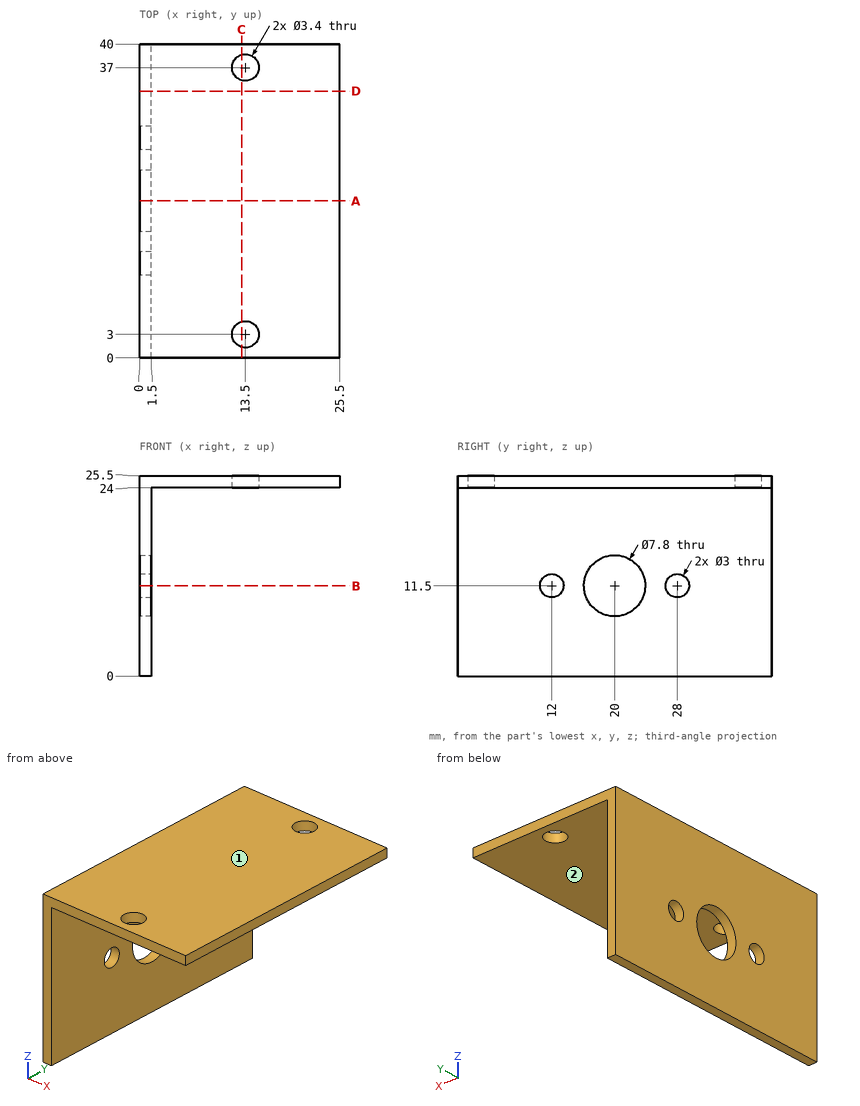
The drawing under review shows one solid part. Ordinate dimensions are in mm from its lowest x, y, z. A direction names the side the tool comes from. Round coordinates to 2 decimals unless told otherwise and drop trailing zeros. Write each loop counter-clockwise with the first axis right and the second up, starting at its lowest first coordinate (ties: lowest second). Pieces come first, ordered by that corner, then holes. Notation, with made-up numbers: (63, 58.25) - (115, 58.25) arc R16 cw to (115, 81.25) - close; hole circle Ø8 at (-4.5, 49.25). An arc over 180 degrees is marked (long way). One line per question, with ' | ' between items.
Item 1: For P1, Ø9, axis at y = 20, z = 11.5, coming from the +X side; P2, Ø1.5, axis at x = 13, y = 21.5, coming from the -Z side; P3, Ø10, axis at x = 9.5, z = 11.5, coming from the -Y side, all flat-tipped, find the tip position at first contact; note any pin that passes through.
Resolved:
P1: stops at x = 1.5 | P2: stops at z = 24 | P3: passes through
Item 2: Add section C-C, the plane x = 13. Give the boundary of the cut face in (y, z).
Resolved:
outline: (0, 24) - (1.38, 24) - (1.38, 25.5) - (0, 25.5) - close; (4.62, 24) - (35.38, 24) - (35.38, 25.5) - (4.62, 25.5) - close; (38.62, 24) - (40, 24) - (40, 25.5) - (38.62, 25.5) - close
Item 3: To check wall thickness, follow probe 1 along Y at (x, z) = (13.5, 24.7); probe 2 along Y at (x, z) = (0.8, 11.5); probe 3 along X at (y, z) = (29.5, 12.25). State the ranges of each line that lie inside material, in increasing order.
Resolved:
probe 1: y = 0 to 1.3, 4.7 to 35.3, 38.7 to 40 | probe 2: y = 0 to 10.5, 13.5 to 16.1, 23.9 to 26.5, 29.5 to 40 | probe 3: x = 0 to 1.5
Item 4: Add section D-D, the plane y = 34. Give the boundary of the cut face in (x, z), then the cut area to 4 significant figures.
Resolved:
outline: (0, 0) - (1.5, 0) - (1.5, 24) - (25.5, 24) - (25.5, 25.5) - (0, 25.5) - close | area: 74.25 mm2
Item 5: Add section A-A, the plane y = 20. Give the boundary of the cut face in (x, z), then the cut area to 4 significant figures.
Resolved:
outline: (0, 0) - (1.5, 0) - (1.5, 7.6) - (0, 7.6) - close; (0, 15.4) - (1.5, 15.4) - (1.5, 24) - (25.5, 24) - (25.5, 25.5) - (0, 25.5) - close | area: 62.55 mm2
Item 6: Add section B-B, the plane z = 11.5. Give the boundary of the cut face in (x, y), then the cut area to 3 significant figures.
Resolved:
outline: (0, 0) - (1.5, 0) - (1.5, 10.5) - (0, 10.5) - close; (0, 13.5) - (1.5, 13.5) - (1.5, 16.1) - (0, 16.1) - close; (0, 23.9) - (1.5, 23.9) - (1.5, 26.5) - (0, 26.5) - close; (0, 29.5) - (1.5, 29.5) - (1.5, 40) - (0, 40) - close | area: 39.3 mm2
Item 7: For the marked faces 1 and 2, list the 3-axis set-ups (+Z, -Z, +X, -X, +Y, -Y) from which the entire face can be reached by the end or side of a thin tool; tool diameter is ignored.
Resolved:
face 1: +Z, +X, -X, +Y, -Y | face 2: -Z, +X, +Y, -Y
